Could you check a few things on this model? Use its own coordinates, in mm. Face numbers are marked on the shaded views. A direction names the side the tool comes from. Give positions to 0.01 mm unless a question says otherwise; leave off trailing zeros. Loops run counter-clockwise (first coordinate to the right, second up) from the corner with the lowest first, then second, coordinate; pieces in that order, holes last. Notation, with made-up numbers: (81, 10.5) - (123, 10.5) arc R22 cw to (123, 47.5) - close; hole circle Ø4 at (-6.5, 64.25). An arc over 180 degrees is marked (long way). Use CSV: the item, a comma, the result in double quotes.
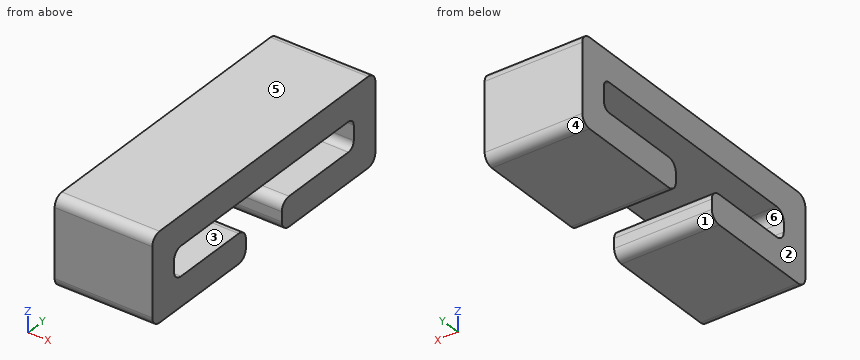
Autodesk Inventor part; units mm, degrees
ref_plane "YZ Plane" through (0, 0, 0) normal (1, 0, 0) x (0, 1, 0)
ref_plane "XZ Plane" through (0, 0, 0) normal (0, 1, 0) x (-1, 0, 0)
ref_plane "XY Plane" through (0, 0, 0) normal (0, 0, 1) x (1, 0, 0)
sketch "Эскиз1" plane through (0, 0, 0) normal (1, 0, 0) x (0, 1, 0)
  line L0 (-0.75, 0) -> (-24, 0)
  line L1 (-25, -1) -> (-25, -2)
  line L2 (0, -2.25) -> (0, -0.75)
  line L3 (2, 3) -> (-27, 3)
  line L4 (-28, 2) -> (-28, -5)
  line L5 (3, -5) -> (3, 2)
  line L6 (-15, -4) -> (-15, -5)
  line L7 (-10, -5) -> (-10, -4)
  arc A0 (2, -6) -> (3, -5) centre (2, -5) ccw
  arc A1 (3, 2) -> (2, 3) centre (2, 2) ccw
  arc A2 (-27, 3) -> (-28, 2) centre (-27, 2) ccw
  arc A3 (-28, -5) -> (-27, -6) centre (-27, -5) ccw
  arc A4 (-25, -2) -> (-24, -3) centre (-24, -2) ccw
  arc A5 (-24, 0) -> (-25, -1) centre (-24, -1) ccw
  arc A6 (0, -0.75) -> (-0.75, 0) centre (-0.75, -0.75) ccw
  arc A7 (-0.75, -3) -> (0, -2.25) centre (-0.75, -2.25) ccw
  line L8 (-0.4776, -6) -> (-9, -6)
  line L9 (-16, -6) -> (-17.3462, -6)
  line L10 (-24, -3) -> (-16, -3)
  line L11 (-9, -3) -> (-0.75, -3)
  line L12 (-27, -6) -> (-16, -6)
  line L13 (-9, -6) -> (2, -6)
  arc A8 (-9, -3) -> (-10, -4) centre (-9, -4) ccw
  arc A9 (-10, -5) -> (-9, -6) centre (-9, -5) ccw
  arc A10 (-15, -4) -> (-16, -3) centre (-16, -4) ccw
  arc A11 (-16, -6) -> (-15, -5) centre (-16, -5) ccw
  line L14 (2, -5) -> (-27, 2) construction
  line L15 (2, 2) -> (-27, -5) construction
  line L16 (-10, -4) -> (3, -4) construction
  line L17 (-15, -4) -> (-28, -4) construction
  point P0 (0, 0)
  point P1 (-25, -3)
  point P2 (-25, 0)
  point P3 (0, -3)
  dimension "d1" = 3
  dimension "d4" = 3
  dimension "d5" = 3
  dimension "d6" = 3
  dimension "d7" = 5
  dimension "d8" = 1
  dimension "d9" = 0.75
  dimension "d10" = 13
  dimension "d11" = 1
  dimension "d12" = 1
  dimension "d15" = 3
  dimension "d16" = 25
extrude "Выдавливание1" add sketch "Эскиз1" along normal blind 10
properties part number "_3DПЕЧАТЬ"
1) Suppose I cut it at A-A (y = -17). Please give me the cut outline in (x, z).
Answer below:
outline,"(0, -6) - (10, -6) - (10, -3) - (0, -3) - close; (0, 0) - (10, 0) - (10, 3) - (0, 3) - close"
2) I need wall thicknesses on line 1 along Y through (x, z) = (7.75, -1.5); line 2 along Z through (x, y) = (8.5, -20.5); line 3 along Y through (x, z) = (4.5, -4.25). Which ranges of each line are inside material? Lowest first, please.
Answer below:
line 1,"y = -28 to -25, 0 to 3"
line 2,"z = -6 to -3, 0 to 3"
line 3,"y = -28 to -15, -10 to 3"
3) Which directions (+Z, -Z, +X, -X, +Y, -Y) give clear straight access to the entire face, cutting with the end or side of a thin tool? Please do the marked faces 1, 2 and 3.
Answer below:
face 1,"-Z, +X, -X"
face 2,"+Z, -Z, -X, +Y, -Y"
face 3,"+X, -X"
4) Suppose I cut it at C-C (x = 3). Please give me the cut outline in (y, z), plus the area to 3 significant figures.
Answer below:
outline,"(-28, -5) arc R1 ccw to (-27, -6) - (-16, -6) arc R1 ccw to (-15, -5) - (-15, -4) arc R1 ccw to (-16, -3) - (-24, -3) arc R1 cw to (-25, -2) - (-25, -1) arc R1 cw to (-24, 0) - (-0.75, 0) arc R0.75 cw to (0, -0.75) - (0, -2.25) arc R0.75 cw to (-0.75, -3) - (-9, -3) arc R1 ccw to (-10, -4) - (-10, -5) arc R1 ccw to (-9, -6) - (2, -6) arc R1 ccw to (3, -5) - (3, 2) arc R1 ccw to (2, 3) - (-27, 3) arc R1 ccw to (-28, 2) - close"
area,"188 mm2"
5) Suppose I cut it at D-D (y = -12.5). Please give me the cut outline in (x, z), plus the area to 3 significant figures.
Answer below:
outline,"(0, 0) - (10, 0) - (10, 3) - (0, 3) - close"
area,"30.0 mm2"
6) We'd pull the mould along Y, two halves only. Please class the marked faces 4, 5 and 6: +Y half, -Y half, draft (parallel to the pull), parting line (faces both ways), or undercut.
Answer below:
face 4,"+Y half"
face 5,"draft"
face 6,"undercut"
7) Suppose I cut it at B-B (z = -4.5). Please give me the cut outline in (x, y).
Answer below:
outline,"(0, -28) - (10, -28) - (10, -15) - (0, -15) - close; (0, -10) - (10, -10) - (10, 3) - (0, 3) - close"
